```python
from build123d import *

# Parameters (mm, degrees)
SALIENTE_EXTRUIR1_DEPTH = 29
CORTAR_EXTRUIR1_DEPTH   = 14.5
CHAFL_N1_SIZE           = 1
CROQUIS3_R              = 0.5
CORTAR_EXTRUIR2_DEPTH   = 1
CROQUIS4_R              = 0.5
CORTAR_EXTRUIR3_DEPTH   = 1
CORTAR_EXTRUIR5_DEPTH   = 0.2


with BuildPart() as part:
    # Croquis1 → Saliente-Extruir1 (new body)
    with BuildSketch(Plane(origin=(0, 0, 0), x_dir=(0, 0, -1), z_dir=(1, 0, 0))):
        with BuildLine():
            Line((0, 0), (15, 0))
            Line((15, 0), (12.757359313, 2.242640687))
            ThreePointArc((12.757359313, 2.242640687), (12.108512615, 2.67618619), (11.343145751, 2.828427125))
            Line((11.343145751, 2.828427125), (0, 2.828427125))
            ThreePointArc((0, 2.828427125), (-3.414213562, 1.414213562), (0, 0))
        make_face()
    extrude(amount=SALIENTE_EXTRUIR1_DEPTH)

    # Croquis2 → Cortar-Extruir1 (cut, symmetric)
    with BuildSketch(Plane(origin=(0, 2.828427125, 0), x_dir=(1, 0, 0), z_dir=(0, 1, 0))):
        Polygon((2, 0), (2, 11.343145751), (27, 11.343145751), (27, 0), (27, -11.34659481), (2, -9.45811087), align=None)
    extrude(amount=CORTAR_EXTRUIR1_DEPTH, both=True, mode=Mode.SUBTRACT)

    # Chaflán1
    chafl_n1_edges = [part.edges().sort_by_distance(p)[0] for p in [
        (14.5, 0, -11.343145751),
    ]]
    chamfer(chafl_n1_edges, length=CHAFL_N1_SIZE)

    # Croquis3 → Cortar-Extruir2 (cut)
    with BuildSketch(Plane.ZY.offset(-27)):
        with Locations((1.414213562, 1.414213562)):
            Circle(CROQUIS3_R)
    extrude(amount=-CORTAR_EXTRUIR2_DEPTH, mode=Mode.SUBTRACT)

    # Croquis4 → Cortar-Extruir3 (cut)
    with BuildSketch(Plane(origin=(2, 0, 0), x_dir=(0, 0, -1), z_dir=(1, 0, 0))):
        with Locations((-1.414213562, 1.414213562)):
            Circle(CROQUIS4_R)
    extrude(amount=-CORTAR_EXTRUIR3_DEPTH, mode=Mode.SUBTRACT)

    # Croquis5 → Cortar-Extruir5 (cut)
    with BuildSketch(Plane(origin=(0, 2.85, 0), x_dir=(1, 0, 0), z_dir=(0, 1, 0))):
        with BuildLine():
            Line((13.15, 11.343145751), (15.85, 11.343145751))
            ThreePointArc((15.85, 11.343145751), (14.5, 12.693145751), (13.15, 11.343145751))
        make_face()
    extrude(amount=-CORTAR_EXTRUIR5_DEPTH, mode=Mode.SUBTRACT)


solid = part.part
```
Work out the finished part from the listing and answer in its coordinate system (mm). A direction names the side the tool comes from. Give positions to 0.01 mm unless a question says otherwise; leave off trailing zeros. Loops run counter-clockwise (first coordinate to the right, second up) from the corner with the lowest first, then second, coordinate; pieces in that order, holes last. Notation, with made-up numbers: (-35, 45.25) - (4, 45.25) arc R13 cw to (4, 50.25) - close; hole circle Ø8 at (46.25, -6). An arc over 180 degrees is marked (long way). Use CSV: the item, a comma, the result in double quotes. Start each with the question number.
(1) Determine the mould class of faces 5 (the face through (28, 1.4, 1.4)), 6 (the face through (1, 1.4, 1.4)), 7 (the face through (0, 1, -6)), 8 (the face through (14.325, 0.507, -11.836)) for opening direction Y: released by +Y, released by -Y, zero draft, split by the parting line, or undercut.
(2) Find section B-B, the plane x = 21.25. Determine the outline of the cut face in (y, z), plus the area to 3 significant figures.
(3) Each of these flat-tipped pins is pushed along its axis until it touches: pin 1 (1.1 mm diameter, centred on y = 1.5, z = 1.5, fed in from -X); pin 2 (1.5 mm diameter, centred on x = 16.5, y = 2, fed in from +Z); pin 3 (1 mm diameter, centred on x = 11.5, z = -11.5, fed in from +Y); pin 4 (7.5 mm diameter, centred on x = 17, z = -9, fed in from -Y). Where does it stop, or does it pass through?
(4) Find section A-A, the plane z = -11. Determine the outline of the cut face in (x, y).
(5) Find the intervals of material crossed by L1, parallel to X at y = 2, z = -5.25; L2, parallel to Y at x = 27.5, z = -10.75; L3, parallel to Z at x = 10, y = 1.45, in increasing order.
(6) A tool of negligible diameter and unlimited length cuts with its end or side. For faces 1 (the face through (1, 2.828, -6)), 2 (the face through (1.507, 1.223, 0.952)), 3 (the face through (14, 0, -14)), 4 (the face through (14, 2, -11.343)), from which of +Z, -Z, +X, -X, +Y, -Y can it reach the whole face along a straight path? Write none if from no direction.
Results found:
1,face 5,"undercut"
1,face 6,"undercut"
1,face 7,"zero draft"
1,face 8,"released by -Y"
2,outline,"(0, -15) - (2.24, -12.76) arc R2 ccw to (2.83, -11.34) - (1, -11.34) - (0, -12.34) - close"
2,area,"5.76 mm^2"
3,pin 1,"x = 0"
3,pin 2,"z = -11.34"
3,pin 3,"y = 2.83"
3,pin 4,"y = 0"
4,outline,"(0, 0) - (2, 0) - (2, 2.83) - (0, 2.83) - close; (27, 0) - (29, 0) - (29, 2.83) - (27, 2.83) - close"
5,L1,"0 to 2, 27 to 29"
5,L2,"0 to 2.83"
5,L3,"-13.55 to -11.34"
6,face 1,"-Z, +X, -X, +Y"
6,face 2,"none"
6,face 3,"-Z, +X, -X, -Y"
6,face 4,"+Z, +Y, -Y"
